Geometry check sheet. Reference: the model listing, model coordinates, mm. A direction names the side the tool comes from. Round coordinates to 2 decimals unless told otherwise and drop trailing zeros. Loops run counter-clockwise (first coordinate to the right, second up) from the corner with the lowest first, then second, coordinate; pieces in that order, holes last. Notation, with made-up numbers: M -9.75,84 L 2.25,84 A25 ccw 2.25,106 Z; hole C 77.5,17 d11. An arc over 180 degrees is marked long. Use one line per item in the form item = value. Start each with the question number.
1. Material ranges on line 1 (Y direction, x = 3.5, z = 30.5); line 2 (Z direction, x = 25, y = -11.75); line 3 (Z direction, x = 28, y = 8), recorded low to high.
2. Go/stop test with flat-tipped pins: pin 1 (5.5 mm diameter, centred on x = 18.5, z = 19.5, fed in from -Y); pin 2 (14.5 mm diameter, centred on x = 23, y = -7.5, fed in from +Z); pin 3 (10 mm diameter, centred on y = 5, z = 21, fed in from +X); pin 4 (1.5 mm diameter, centred on x = 32.5, z = 25, fed in from -Y). Record where each tip stops, or that it passes through.
3. Cross-section at D-D (z = 11). Record the boundary of the cut face in (x, y).
4. Set-up check for faces 1 (the flat face through (15, -7, 12.7)), 2 (the flat face through (38.1, 6, 6)): record each of +Z, -Z, +X, -X, +Y, -Y from which the full face is reachable in a straight line by a thin tool's end or side.
5. Cross-section at C-C (z = 22). Record the boundary of the cut face in (x, y).
6. Cross-section at B-B (y = 2). Record the boundary of the cut face in (x, z).
7. Cross-section at A-A (x = 8). Record the boundary of the cut face in (y, z).
```python
from build123d import *

# Parameters (mm, degrees)
F0_W     = 25.4
F0_H     = 31.75
F1_DEPTH = 38.1
F2_W     = 13.111336
F2_H     = 19.05
F3_DEPTH = 38.101
F5_DEPTH = 12.289664
F7_DEPTH = 25.4


with BuildPart() as f1:
    # F0 (on Right) → F1 (new body)
    with BuildSketch(Plane.YZ):
        with Locations((-0.411336, 15.875)):
            Rectangle(F0_W, F0_H)
    extrude(amount=F1_DEPTH)

    # F2 (on face) → F3 (cut, through all)
    with BuildSketch(Plane.YZ.offset(38.1)):
        with Locations((-6.555668, 22.225)):
            Rectangle(F2_W, F2_H)
    extrude(amount=-F3_DEPTH, mode=Mode.SUBTRACT)

    # F4 (on face) → F5 (cut, through all)
    with BuildSketch(Plane.XZ):
        Polygon((25.4, 31.75), (38.1, 12.7), (38.1, 31.75), align=None)
    extrude(amount=-F5_DEPTH, mode=Mode.SUBTRACT)

    # F6 (on face) → F7 (cut)
    with BuildSketch(Plane.XY.offset(12.7)):
        Polygon((38.1, -13.111336), (38.1, 0), (25.4, -13.111336), align=None)
    extrude(amount=-F7_DEPTH, mode=Mode.SUBTRACT)


solid = f1.part
```
Reported:
q1.line_1 = 0 to 12.29
q1.line_2 = 0 to 12.7
q1.line_3 = 0 to 27.85
q2.pin_1 = 0
q2.pin_2 = 12.7
q2.pin_3 = 35.9
q2.pin_4 = through
q3.outline = M 0,-13.11 L 25.4,-13.11 L 38.1,0 L 38.1,12.29 L 0,12.29 Z
q4.face_1 = +Z, +X, -X, -Y
q4.face_2 = +Z, -Z, +X, +Y, -Y
q5.outline = M 0,0 L 31.9,0 L 31.9,12.29 L 0,12.29 Z
q6.outline = M 0,0 L 38.1,0 L 38.1,12.7 L 25.4,31.75 L 0,31.75 Z
q7.outline = M -13.11,0 L 12.29,0 L 12.29,31.75 L 0,31.75 L 0,12.7 L -13.11,12.7 Z
